Here's how the part is built. I have some questions about the finished solid (model axes, mm). Coordinates: 2 decimals unless noted, no trailing zeros. Loops run counter-clockwise (first coordinate to the right, second up) from the corner with the lowest first, then second, coordinate; pieces in that order, holes last. Notation, with made-up numbers: (59, -38.75) - (117, -38.75) arc R21 ccw to (117, -4.75) - close; hole circle Ø2 at (44, 25.5). An arc over 180 degrees is marked (long way). Use a Markdown table: item, result.
```python
from build123d import *

# Parameters (mm, degrees)
CROQUIS2_R     = 3.572
EXTRUIR1_DEPTH = 12.358
CROQUIS3_R     = 3.572
EXTRUIR2_DEPTH = 12.358


with BuildPart() as part:
    # Croquis1 → Revolución1 (revolve)
    with BuildSketch(Plane.XY):
        with BuildLine():
            Line((5.214, 19.4), (5.214, 11.2))
            ThreePointArc((5.214, 11.2), (5.272578644, 11.058578644), (5.414, 11))
            Line((5.414, 11), (8.586, 11))
            ThreePointArc((8.586, 11), (8.727421356, 11.058578644), (8.786, 11.2))
            Line((8.786, 11.2), (8.786, 19.4))
            ThreePointArc((8.786, 19.4), (8.610264069, 19.824264069), (8.186, 20))
            Line((8.186, 20), (5.814, 20))
            ThreePointArc((5.814, 20), (5.389735931, 19.824264069), (5.214, 19.4))
        make_face()
    revolve(axis=Axis((50, 0, 0), (-1, 0, 0)))

    # Croquis2 → Extruir1 (cut)
    with BuildSketch(Plane(origin=(0, 0, 0), x_dir=(0, 0, -1), z_dir=(1, 0, 0))):
        with Locations((0, 15)):
            Circle(CROQUIS2_R)
    extrude(amount=EXTRUIR1_DEPTH, mode=Mode.SUBTRACT)

    # Croquis3 → Extruir2 (cut)
    with BuildSketch(Plane(origin=(0, 0, 0), x_dir=(0, 0, -1), z_dir=(1, 0, 0))):
        with Locations((0, -15)):
            Circle(CROQUIS3_R)
    extrude(amount=EXTRUIR2_DEPTH, mode=Mode.SUBTRACT)


solid = part.part
```
Q1. If we mould it in two halves opening along Z, with no side actions, what happens to faces 1 (the face through (8.786, -8.4, 8.4)), 2 (the face through (6.97, 18.54, 0.47)), 3 (the face through (6.983, -4.336, 19.524))? For each: pulls with the +Z half, pulls with the -Z half, needs draft (parallel to the pull), parting line crosses it, or undercut.
Check values:
| item | result |
|---|---|
| face 1 | needs draft |
| face 2 | undercut |
| face 3 | parting line crosses it |
Q2. Please list where these lines run through material, in increasing order: L1, parallel to Y at x = 7.3, z = 0; L2, parallel to Y at x = 5.55, z = 3; L3, parallel to Z at x = 6.25, y = 0. Write a range as from..to.
Check values:
| item | result |
|---|---|
| L1 | -20..-18.57, -11.43..-11, 11..11.43, 18.57..20 |
| L2 | -19.71..-16.94, -13.06..-10.58, 10.58..13.06, 16.94..19.71 |
| L3 | -20..-11, 11..20 |
Q3. I want a section at C-C, the plane x = 6.65. Write out the boundary of the cut face in (y, z).
Check values:
| item | result |
|---|---|
| outline | circle Ø40 at (0, 0); hole circle Ø7.14 at (-15, 0); hole circle Ø22 at (0, 0); hole circle Ø7.14 at (15, 0) |
Q4. I want a section at A-A, the plane y = 0. Write out the boundary of the cut face in (x, z).
Check values:
| item | result |
|---|---|
| outline | (5.21, -19.4) arc R0.6 ccw to (5.81, -20) - (8.19, -20) arc R0.6 ccw to (8.79, -19.4) - (8.79, -11.2) arc R0.2 ccw to (8.59, -11) - (5.41, -11) arc R0.2 ccw to (5.21, -11.2) - close; (5.21, 11.2) arc R0.2 ccw to (5.41, 11) - (8.59, 11) arc R0.2 ccw to (8.79, 11.2) - (8.79, 19.4) arc R0.6 ccw to (8.19, 20) - (5.81, 20) arc R0.6 ccw to (5.21, 19.4) - close |
Q5. I want a section at B-B, the plane z = 0. Write out the boundary of the cut face in (x, y), then the cut area to 3 significant figures.
Check values:
| item | result |
|---|---|
| outline | (5.21, -19.4) arc R0.6 ccw to (5.81, -20) - (8.19, -20) arc R0.6 ccw to (8.79, -19.4) - (8.79, -18.57) - (5.21, -18.57) - close; (5.21, -11.43) - (8.79, -11.43) - (8.79, -11.2) arc R0.2 ccw to (8.59, -11) - (5.41, -11) arc R0.2 ccw to (5.21, -11.2) - close; (5.21, 11.2) arc R0.2 ccw to (5.41, 11) - (8.59, 11) arc R0.2 ccw to (8.79, 11.2) - (8.79, 11.43) - (5.21, 11.43) - close; (5.21, 18.57) - (8.79, 18.57) - (8.79, 19.4) arc R0.6 ccw to (8.19, 20) - (5.81, 20) arc R0.6 ccw to (5.21, 19.4) - close |
| area | 12.9 mm^2 |
